```python
from build123d import *

# Parameters (mm, degrees)
F1_DEPTH = 15
F0_W     = 26.8
F0_H     = 30
F2_DEPTH = 1.6


# Not quite as in the source:
# - a feature names something its author has since deleted; it is built from what else it names


with BuildPart() as f1:
    # F0 (on Top) → F1 (new body)
    with BuildSketch(Plane.XY):
        with BuildLine():
            ThreePointArc((30, -15), (25.6066017178, -4.3933982822), (15, 0))
            ThreePointArc((15, 0), (4.3933982822, -4.3933982822), (0, -15))
            Line((0, -15), (0, -45))
            Line((0, -45), (1.6, -45))
            Line((1.6, -45), (1.6, -15))
            ThreePointArc((1.6, -15), (15, -1.6), (28.4, -15))
            Line((28.4, -15), (28.4, -45))
            Line((28.4, -45), (30, -45))
            Line((30, -45), (30, -15))
        make_face()
        with BuildLine():
            Line((1.6, -45), (0, -45))
            ThreePointArc((0, -45), (4.3933982822, -55.6066017178), (15, -60))
            ThreePointArc((15, -60), (25.6066017178, -55.6066017178), (30, -45))
            Line((30, -45), (28.4, -45))
            ThreePointArc((28.4, -45), (15, -58.4), (1.6, -45))
        make_face()
    extrude(amount=F1_DEPTH)

    # F0 (on Top) → F2 (join)
    with BuildSketch(Plane.XY):
        with BuildLine():
            ThreePointArc((28.4, -15), (15, -1.6), (1.6, -15))
            Line((1.6, -15), (28.4, -15))
        make_face()
        with BuildLine():
            Line((28.4, -45), (1.6, -45))
            ThreePointArc((1.6, -45), (15, -58.4), (28.4, -45))
        make_face()
        with Locations((15, -30)):
            Rectangle(F0_W, F0_H)
    extrude(amount=F2_DEPTH)


solid = f1.part
```
Can you work these out from the model? Positions are in its coordinate system, mm. A direction names the side the tool comes from. Coordinates: 2 decimals unless noted, no trailing zeros. Order: outer loops, then holes, each group sorted by start corner. A loop starts at its lowest first (then second) coordinate and runs counter-clockwise, first axis right, second up.
1. If we section it at B-B (y = -19): Please give me the cut outline in (x, z).
2. I'm going to push flat-ended pins straight in: pin 1 (3 mm diameter, centred on x = 4, z = 13, fed in from -Y); pin 2 (3 mm diameter, centred on x = 19.5, y = -18, fed in from +Z). Where does each tip first touch, or does it pass through?
3. If we section it at C-C (x = 15): Please give me the cut outline in (y, z).
4. If we section it at A-A (z = 3.25): Please give me the cut outline in (x, y).
5. I need wall thicknesses on line 1 (X direction, y = -33, z = 13); line 2 (Z direction, x = 18.5, y = -7); line 3 (X direction, y = -55, z = 6.75). Which ranges of each line are inside material? Lowest first, please.
6. Thinking about a two-plate mould opening in Y: for faces 3 (the face through (15, 0, 7)), 4 (the face through (14.705, -1.603, 8.206)), 5 (the face through (30, -30, 7)), 6 (the face through (15, -30, 1.6)), which applies, +Y half, -Y half, draft (parallel to the pull), parting line (faces both ways), or undercut?
7. For faces 1 (the face through (1.6, -30, 8)), 2 (the face through (15, -60, 7)), which set-ups out of +Z, -Z, +X, -X, +Y, -Y let a thin tool reach every point of the face, with its end or its side?
Entries:
1. outline: (0, 0) - (30, 0) - (30, 15) - (28.4, 15) - (28.4, 1.6) - (1.6, 1.6) - (1.6, 15) - (0, 15) - close
2. pin 1: stops at y = -56.61
2. pin 2: stops at z = 1.6
3. outline: (-60, 0) - (0, 0) - (0, 15) - (-1.6, 15) - (-1.6, 1.6) - (-58.4, 1.6) - (-58.4, 15) - (-60, 15) - close
4. outline: (0, -45) arc R15 ccw to (30, -45) - (30, -15) arc R15 ccw to (0, -15) - close; hole (1.6, -45) arc R13.4 ccw to (28.4, -45) - (28.4, -15) arc R13.4 ccw to (1.6, -15) - close
5. line 1: x = 0 to 1.6, 28.4 to 30
5. line 2: z = 0 to 1.6
5. line 3: x = 3.82 to 6.08, 23.92 to 26.18
6. face 3: +Y half
6. face 4: undercut
6. face 5: draft
6. face 6: undercut
7. face 1: +Z
7. face 2: +Z, -Z, -Y
